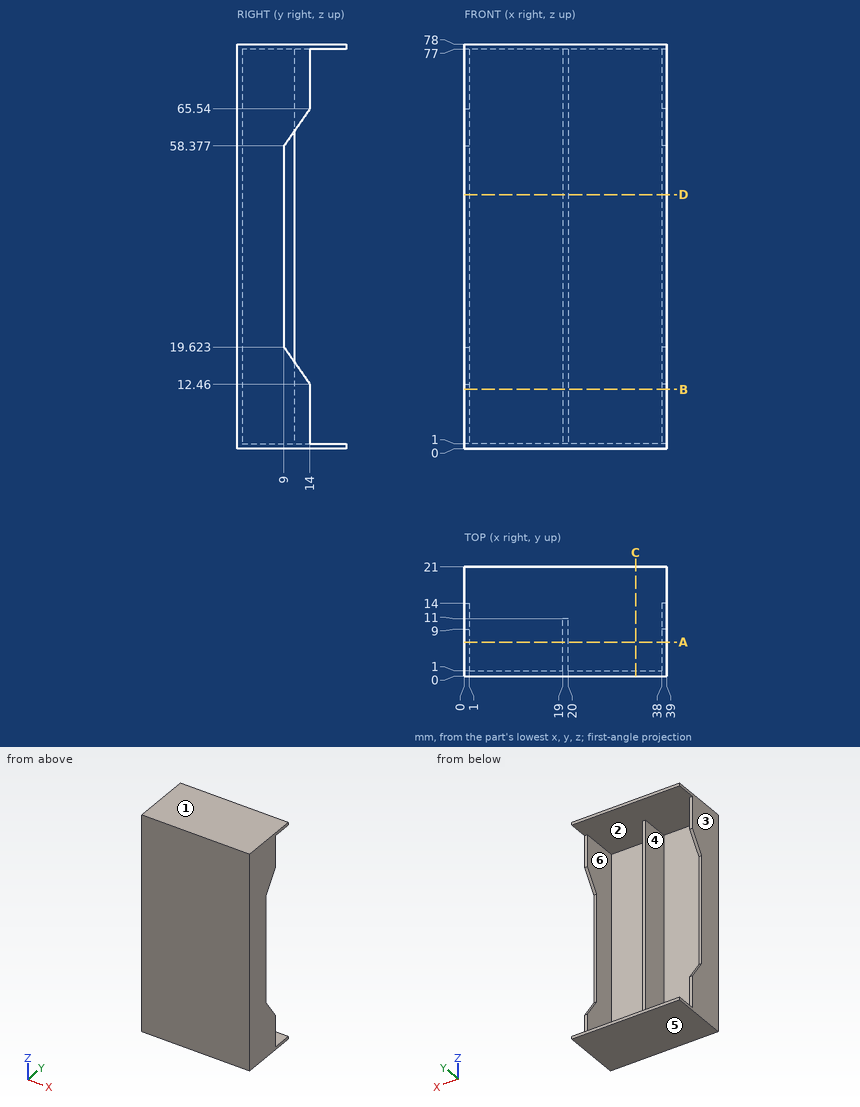
Check sheet for the drawn part. Datum: minimum x, y, z corner. Units: mm. A direction names the side the tool comes from. Give positions to 0.01 mm unless a question says otherwise; leave off trailing zeros. Order: outer loops, then holes, each group sorted by start corner. A loop starts at its lowest first (then second) coordinate and runs counter-clockwise, first axis right, second up. Notation, with made-up numbers: (-8, 23) -> (1, 23) arc R35 cw to (1, 57) -> close; hole circle Ø8 at (76.5, -6). An arc over 180 degrees is marked (long way). One line per item, written item: value.
(1) Sectioned sample at B-B on z = 11.5. Record the cut outline in (x, y).
Final values:
outline: (0, 0) -> (39, 0) -> (39, 14) -> (38, 14) -> (38, 1) -> (20, 1) -> (20, 11) -> (19, 11) -> (19, 1) -> (1, 1) -> (1, 14) -> (0, 14) -> close
(2) Draft check along X on the marked faces 3, 4, 5 and 6. Enter one of: pulls with the +X half, pulls with the -X half, needs draft (parallel to the pull), parting line crosses it, or undercut.
Final values:
face 3: pulls with the -X half
face 4: undercut
face 5: needs draft
face 6: undercut
(3) Tool access check on the marked faces 1 and 2. Record the directions out of +Z, -Z, +X, -X, +Y, -Y that give a thin tool (end or side, any length) a straight path to the whole face; none if there is none.
Final values:
face 1: +Z, +X, -X, +Y, -Y
face 2: +Y
(4) Gauge pin test, flat ends, axial feed: pin 1 (0.8 mm diameter, centred on x = 0.5, z = 5.5, fed in from +Y); pin 2 (5 mm diameter, centred on x = 16, z = 27, fed in from +Y); pin 3 (1.1 mm diameter, centred on x = 19.5, z = 54.5, fed in from +Y). Record the tip position at first contact, or that the pin passes through.
Final values:
pin 1: y = 14
pin 2: y = 1
pin 3: y = 11
(5) Scan lines: line 1 along X through (y, z) = (2.5, 48.5); line 2 along X through (y, z) = (12.25, 14); line 3 along Z through (x, y) = (12.5, 8). Record each from-to range of solid material in increasing order. Write a range as [from, to].
Final values:
line 1: [0, 1], [19, 20], [38, 39]
line 2: [0, 1], [38, 39]
line 3: [0, 1], [77, 78]
(6) Sectioned sample at C-C on x = 33. Record the cut outline in (y, z), then the cut area to 3 significant figures.
Final values:
outline: (0, 0) -> (21, 0) -> (21, 1) -> (1, 1) -> (1, 77) -> (21, 77) -> (21, 78) -> (0, 78) -> close
area: 118 mm^2
(7) Sectioned sample at D-D on z = 49. Record the cut outline in (x, y).
Final values:
outline: (0, 0) -> (39, 0) -> (39, 9) -> (38, 9) -> (38, 1) -> (20, 1) -> (20, 11) -> (19, 11) -> (19, 1) -> (1, 1) -> (1, 9) -> (0, 9) -> close
(8) Sectioned sample at A-A on y = 6.5. Record the cut outline in (x, z), then the cut area to 3 significant figures.
Final values:
outline: (0, 0) -> (39, 0) -> (39, 78) -> (0, 78) -> close; hole (1, 1) -> (19, 1) -> (19, 77) -> (1, 77) -> close; hole (20, 1) -> (38, 1) -> (38, 77) -> (20, 77) -> close
area: 306 mm^2
